Verification items for this drawing (mm, ordinates from the low corner). A direction names the side the tool comes from. Coordinates: 2 decimals unless noted, no trailing zeros. Loops run counter-clockwise (first coordinate to the right, second up) from the corner with the lowest first, then second, coordinate; pieces in that order, holes last. Notation, with made-up numbers: (80.5, -32) - (139.5, -32) arc R19 ccw to (139.5, -17) - close; hole circle Ø9 at (76.5, 63.5). An arc over 180 degrees is marked (long way). One line per item, written item: value. Start each with the question number.
(1) Section check C-C (y = 11). Record the boundary of the cut face in (x, z), plus the area to 3 significant figures.
(2) Draft check along Y on the marked faces 1, 2, 3 and 4. Enter one of: +Y half, -Y half, draft (parallel to the pull), parting line (faces both ways), or undercut.
(3) Section check A-A (x = 22.5). Record the boundary of the cut face in (y, z).
(4) Set-up check for the marked faces 5, 6 and 7: record each of +Z, -Z, +X, -X, +Y, -Y from which the full face is reachable in a straight line by a thin tool's end or side.
(5) Gauge pin test, flat ends, axial feed: P1, Ø2, axis at y = 13.5, z = 31.5, coming from the -X side; P2, Ø1.5, axis at x = 11, z = 22, coming from the -Y side; P3, Ø3.5, axis at x = 11.5, y = 29.5, coming from the +Z side. Record the tip position at first contact, or that the pin passes through.
(6) Section check B-B (z = 14.5). Record the boundary of the cut face in (x, y).
(7) Thickness scan on probe 1 along Y at (x, z) = (22.5, 14); probe 2 along X at (y, z) = (30.5, 17) (1 decimal); probe 3 along X at (y, z) = (26, 31.5) (1 decimal). Record the ranges inside material, lowest first. Write a range as [from, to].
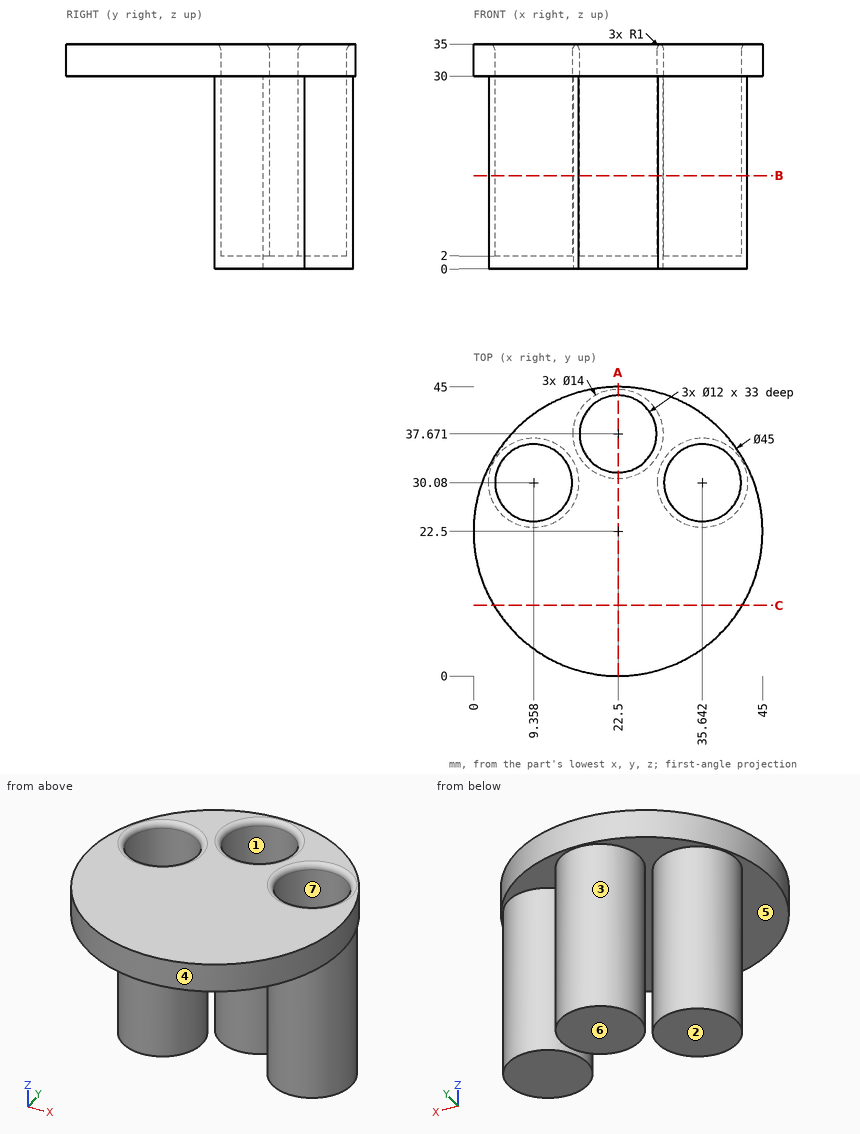
Responses:
1. outline: (3.16, 30) - (41.84, 30) - (41.84, 35) - (3.16, 35) - close
1. area: 193 mm²
2. face 1: undercut
2. face 2: draft
2. face 3: undercut
2. face 4: parting line
3. outline: (0, 30) - (30.67, 30) - (30.67, 0) - (44.67, 0) - (44.67, 30) - (45, 30) - (45, 35) - (44.67, 35) arc R1 ccw to (43.67, 34) - (43.67, 2) - (31.67, 2) - (31.67, 34) arc R1 ccw to (30.67, 35) - (0, 35) - close
4. face 5: -Z
4. face 6: -Z, +X, -X, +Y, -Y
4. face 7: +Z
5. P1: stops at x = 1.47
5. P2: stops at y = 23.14
5. P3: stops at z = 2
6. outline: circle Ø14 at (9.36, 30.08); circle Ø14 at (22.5, 37.67); circle Ø14 at (35.64, 30.08); hole circle Ø12 at (9.36, 30.08); hole circle Ø12 at (22.5, 37.67); hole circle Ø12 at (35.64, 30.08)
7. probe 1: y = [30.67, 31.67], [43.67, 44.67]
7. probe 2: x = [2.4, 3.4], [15.3, 16.3], [28.7, 29.7], [41.6, 42.6]
7. probe 3: x = [0.3, 5], [13.8, 31.2], [40, 44.7]
